```python
from build123d import *

# Parameters (mm, degrees)
BOSS_EXTRUDE1_DEPTH      = 3.81
BOSS_EXTRUDE1_DEPTH_BACK = 2.54
SKETCH6_R                = 6.858
BOSS_EXTRUDE2_DEPTH      = 15.10284
BOSS_EXTRUDE2_TAPER      = 1.783333333
SKETCH9_OUTSIDE_W        = 56.69
SKETCH9_OUTSIDE_H        = 59.144
SKETCH9_OUTSIDE_R        = 5.318470858
CUT_EXTRUDE1_DEPTH       = 15.10284
CUT_EXTRUDE1_TAPER       = 45
SKETCH10_R               = 6.858
BOSS_EXTRUDE3_DEPTH      = 0.13716
SKETCH11_W               = 35.56
SKETCH11_H               = 2.1844


with BuildPart() as part:
    # Sketch1 → Revolve1 (revolve)
    with BuildSketch(Plane(origin=(0, 0, 0), x_dir=(0, 0, -1), z_dir=(1, 0, 0))):
        with BuildLine():
            Line((-17.78, 0), (0, 0))
            Line((0, 0), (0, 4.6228))
            Line((0, 4.6228), (-5.609789755, 4.6228))
            ThreePointArc((-5.609789755, 4.6228), (-5.706991347, 4.642134599), (-5.789394878, 4.697194878))
            Line((-5.789394878, 4.697194878), (-6.64845, 5.55625))
            Line((-6.64845, 5.55625), (-11.88085, 5.55625))
            Line((-11.88085, 5.55625), (-12.803405122, 4.633694878))
            ThreePointArc((-12.803405122, 4.633694878), (-12.885808653, 4.578634599), (-12.983010245, 4.5593))
            Line((-12.983010245, 4.5593), (-14.982324107, 4.5593))
            Line((-14.982324107, 4.5593), (-17.729430508, 2.489206846))
            ThreePointArc((-17.729430508, 2.489206846), (-17.766656664, 2.444447258), (-17.78, 2.387780136))
            Line((-17.78, 2.387780136), (-17.78, 0))
        make_face()
    revolve(axis=Axis((0, 0, 19.812), (0, 0, -1)))

    # Sketch4 → Boss-Extrude1 (add, two sides)
    with BuildSketch(Plane.XY) as boss_extrude1_sk:
        Polygon((0, 9.165435523), (-7.9375, 4.582717762), (-7.9375, -4.582717762), (0, -9.165435523), (7.9375, -4.582717762), (7.9375, 4.582717762), align=None)
    extrude(amount=BOSS_EXTRUDE1_DEPTH)
    extrude(boss_extrude1_sk.sketch, amount=-BOSS_EXTRUDE1_DEPTH_BACK)

    # Sketch5 → Cut-Revolve1 (revolve, cut)
    with BuildSketch(Plane(origin=(0, 0, 0), x_dir=(0, 0, -1), z_dir=(1, 0, 0))):
        Polygon((-3.81, 11.358571047), (2.54, 11.358571047), (2.54, 6.9723), (1.952351108, 9.165435523), (-3.222351108, 9.165435523), (-3.81, 6.9723), align=None)
    revolve(axis=Axis((0, 0, 3.81), (0, 0, -1)), mode=Mode.SUBTRACT)



with BuildPart() as body_2:
    # Sketch6 → Boss-Extrude2 (new body)
    with BuildSketch(Plane.XY.offset(-2.67716)):
        Circle(SKETCH6_R)
    extrude(amount=-BOSS_EXTRUDE2_DEPTH, taper=BOSS_EXTRUDE2_TAPER)

    # Sketch9 outside → Cut-Extrude1 (cut)
    with BuildSketch(Plane(origin=(0, 0, -17.78), x_dir=(-1, 0, 0), z_dir=(0, 0, -1))):
        Rectangle(SKETCH9_OUTSIDE_W, SKETCH9_OUTSIDE_H)
        Circle(SKETCH9_OUTSIDE_R, mode=Mode.SUBTRACT)
    extrude(amount=-CUT_EXTRUDE1_DEPTH, taper=CUT_EXTRUDE1_TAPER, mode=Mode.SUBTRACT)


with BuildPart() as part_1:
    add(part.part)

    add(body_2.part)  # Boss-Extrude3 merges body 2
    # Sketch10 → Boss-Extrude3 (add)
    with BuildSketch(Plane.XY.offset(-2.67716)):
        Circle(SKETCH10_R)
    extrude(amount=BOSS_EXTRUDE3_DEPTH)

    # Sketch11 → Cut-Revolve2 (revolve, cut)
    with BuildSketch(Plane(origin=(0, 0, 0), x_dir=(0, 0, -1), z_dir=(1, 0, 0))):
        with Locations((0, 1.0922)):
            Rectangle(SKETCH11_W, SKETCH11_H)
    revolve(axis=Axis((0, 0, -17.78), (0, 0, 1)), mode=Mode.SUBTRACT)

    # Sketch12 → Cut-Revolve3 (revolve, cut)
    with BuildSketch(Plane(origin=(0, 0, 0), x_dir=(0, 0, -1), z_dir=(1, 0, 0))):
        Polygon((17.78, 0), (-2.289278958, 0), (0, 3.81), (17.78, 3.81), align=None)
    revolve(axis=Axis((0, 0, 17.78), (0, 0, -1)), mode=Mode.SUBTRACT)


solid = part_1.part
```
Input: part model. Units: mm. Frame: model coordinates. A direction names the side the tool comes from. Coordinates: 2 decimals unless noted, no trailing zeros. Loops run counter-clockwise (first coordinate to the right, second up) from the corner with the lowest first, then second, coordinate; pieces in that order, holes last. Notation, with made-up numbers: M 32.5,8 L 85.5,8 A19 ccw 85.5,18 Z; hole C 85.5,86.25 d5. An arc over 180 degrees is marked long. Use a Markdown table: item, result. Add a question column.
1) Line query: L1, parallel to X at y = 0, z = 7.5; L2, parallel to X at y = 0, z = 5; L3, parallel to Y at x = -0.75, z = -3. Output: solid intervals per line, ascending. Write a range as from..to.
2) Section A-A, the plane z = 5. Return the cut outline in (x, y), plus the area to 3 significant figures.
3) Draft query along X for faces 4 (the cylindrical face through (-0.656, 2.084, 9.261)), 5 (the flat face through (-7.938, 0, 1)), 6 (the cylindrical face through (1.67, 5.3, 9.3)), 7 (the flat face through (-4, 1, -17.78)). Return one class per face: +X half, -X half, draft (parallel to the pull), parting line (faces both ways), or undercut.
4) Section B-B, the plane z = 10. Return the cut outline in (x, y).
5) Pin query (flat end, axial travel): P1, Ø1.5, axis at x = 5.5, y = 5, coming from the +Z side; P2, Ø1.5, axis at x = -4.5, z = -5, coming from the +Y side; P3, Ø3, axis at x = 4.5, z = 10, coming from the +Y side; P4, Ø4, axis at x = 0, y = 0, coming from the +Z side. Return the tip coordinate at first contact, or that it passes through.
6) Set-up query: faces 1 (the cylindrical face through (-2.81, -3.67, 4.72)), 2 (the cylindrical face through (-3.72, -0.83, -9.01)), 3 (the flat face through (4.024, 6.842, 0.676)). Return all of +Z, -Z, +X, -X, +Y, -Y with unobstructed straight access to the full face (end or side cutting, diameter ignored); none if empty.
Answer below:
| question | item | result |
|---|---|---|
| 1 | L1 | -5.56..-2.18, 2.18..5.56 |
| 1 | L2 | -4.62..-2.18, 2.18..4.62 |
| 1 | L3 | -6.81..-3.74, 3.74..6.81 |
| 2 | outline | C 0,0 d9.25; hole C 0,0 d4.37 |
| 2 | area | 52.1 mm2 |
| 3 | face 4 | undercut |
| 3 | face 5 | -X half |
| 3 | face 6 | parting line |
| 3 | face 7 | draft |
| 4 | outline | C 0,0 d11.11; hole C 0,0 d4.37 |
| 5 | P1 | z = 3.81 |
| 5 | P2 | y = 5.66 |
| 5 | P3 | y = 4.68 |
| 5 | P4 | through |
| 6 | face 1 | none |
| 6 | face 2 | -Z |
| 6 | face 3 | +Z, -Z, +X, +Y |
